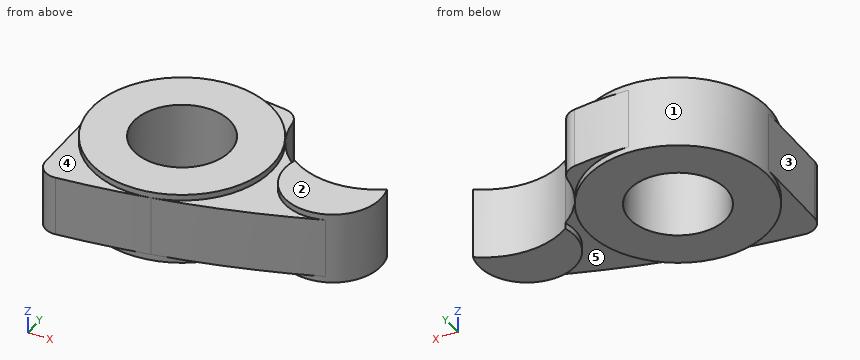
from build123d import *

# Parameters (mm, degrees)
SKETCH_1_R      = 15
SKETCH_1_R_2    = 8
EXTRUDE_1_DEPTH = 6
EXTRUDE_3_DEPTH = 6
EXTRUDE_4_DEPTH = 5


with BuildPart() as part:
    # Sketch 1 → Extrude 1 (new, symmetric)
    with BuildSketch(Plane.XY):
        Circle(SKETCH_1_R)
        Circle(SKETCH_1_R_2, mode=Mode.SUBTRACT)
    extrude(amount=EXTRUDE_1_DEPTH, both=True)



with BuildPart() as body_2:
    # Sketch 2 → Extrude 3 (new, symmetric)
    with BuildSketch(Plane.XY):
        with BuildLine():
            ThreePointArc((17.364190492, 2.386296955), (19.534557037, -5.841997366), (27.889014085, -7.460133888))
            ThreePointArc((27.889014085, -7.460133888), (32.219376902, -3.446824212), (32.617582381, 2.443857334))
            ThreePointArc((32.617582381, 2.443857334), (25, 0), (17.364190492, 2.386296955))
        make_face()
    extrude(amount=EXTRUDE_3_DEPTH, both=True)


with BuildPart() as part_1:
    add(part.part)

    add(body_2.part)  # Extrude 4 merges body 2
    # Sketch 2_4 → Extrude 4 (add, symmetric)
    with BuildSketch(Plane.XY):
        with BuildLine():
            ThreePointArc((15, 0), (11.593101986, -9.51840251), (2.920001822, -14.713041472))
            ThreePointArc((2.920001822, -14.713041472), (15.561957057, -11.62862528), (27.889014085, -7.460133888))
            ThreePointArc((27.889014085, -7.460133888), (19.534557037, -5.841997366), (17.364190492, 2.386296955))
            ThreePointArc((17.364190492, 2.386296955), (15.029800011, 4.466277015), (13.247787509, 7.035348329))
            ThreePointArc((13.247787509, 7.035348329), (14.555356619, 3.625133609), (15, 0))
        make_face()
        with BuildLine():
            ThreePointArc((2.920001822, -14.713041472), (-9.51840251, -11.593101986), (-15, 0))
            Line((-15, 0), (-15, -13.8873794))
            ThreePointArc((-15, -13.8873794), (-14.015653031, -16.10934764), (-11.708571429, -16.873190745))
            ThreePointArc((-11.708571429, -16.873190745), (-4.367649809, -15.973488812), (2.920001822, -14.713041472))
        make_face()
        with BuildLine():
            ThreePointArc((9.245195089, 14.463447909), (4.635046482, 14.946228489), (0, 15))
            ThreePointArc((0, 15), (7.728834811, 12.855547926), (13.247787509, 7.035348329))
            ThreePointArc((13.247787509, 7.035348329), (12.284448117, 9.358081475), (11.777275068, 11.820983737))
            ThreePointArc((11.777275068, 11.820983737), (10.960851201, 13.57305004), (9.245195089, 14.463447909))
        make_face()
    extrude(amount=EXTRUDE_4_DEPTH, both=True)


solid = part_1.part
Could you check a few things on this model? Use its own coordinates, in mm. Face numbers are marked on the shaded views. A direction names the side the tool comes from. Coordinates: 2 decimals unless noted, no trailing zeros. Order: outer loops, then holes, each group sorted by start corner. A loop starts at its lowest first (then second) coordinate and runs counter-clockwise, first axis right, second up.
Q1. Suppose I cut it at D-D on y = -12. Please give me the cut outline in (x, z).
Q2. Will these pins go through, and if not, where does the flat tip stop? pin 1 (2 mm diameter, centred on x = 14, y = -10, fed in from -Z); pin 2 (1 mm diameter, centred on y = 7, z = -3.5, fed in from +X); pin 3 (3 mm diameter, centred on x = 28, z = 4.5, fed in from -Y).
Q3. Suppose I cut it at C-C on x = 11. Please give me the cut outline in (y, z), and give its area (3 significant figures).
Q4. Which directions (+Z, -Z, +X, -X, +Y, -Y) give clear straight access to the entire face, cutting with the end or side of a thin tool? Please do the marked faces 1 and 2.
Q5. Thinking about a two-plate mould opening in X: for the marked faces 3, 4 and 5, which applies, released by +X, released by -X, zero draft, split by the parting line, or undercut?
Q6. Suppose I cut it at B-B on z = -1.25. Please give me the cut outline in (x, y), and give its area (3 significant figures).
Q7. Suppose I cut it at A-A on y = 4.5. Please give me the cut outline in (x, z), and give its area (3 significant figures).
Q8. Please list where these lines run through material, in increasing order: L1, parallel to Z at x = 8.5, y = 14.5; L2, parallel to Y at x = 0, z = -3; L3, parallel to Y at x = 6.5, z = 4.
Answer:
1. outline: (-15, -5) - (-9, -5) - (-9, -6) - (9, -6) - (9, -5) - (14.26, -5) - (14.26, 5) - (9, 5) - (9, 6) - (-9, 6) - (-9, 5) - (-15, 5) - close
2. pin 1: stops at z = -5
2. pin 2: stops at x = 13.55
2. pin 3: stops at y = -7.99
3. outline: (-12.88, -5) - (-10.2, -5) - (-10.2, -6) - (10.2, -6) - (10.2, -5) - (13.53, -5) - (13.53, 5) - (10.2, 5) - (10.2, 6) - (-10.2, 6) - (-10.2, 5) - (-12.88, 5) - close
3. area: 305 mm2
4. face 1: none
4. face 2: +Z, +X, -X, +Y, -Y
5. face 3: released by -X
5. face 4: zero draft
5. face 5: undercut
6. outline: (-15, -13.89) arc R3 ccw to (-11.71, -16.87) arc R150 ccw to (27.89, -7.46) arc R8 ccw to (32.62, 2.44) arc R13.25 cw to (11.78, 11.82) arc R3 ccw to (9.25, 14.46) arc R50 ccw to (0, 15) arc R15 ccw to (-15, 0) - close; hole circle Ø16 at (0, 0)
6. area: 792 mm2
7. outline: (-14.31, -6) - (-6.61, -6) - (-6.61, 6) - (-14.31, 6) - close; (6.61, -6) - (14.31, -6) - (14.31, -5) - (15, -5) - (15, 5) - (14.31, 5) - (14.31, 6) - (6.61, 6) - close
7. area: 192 mm2
8. L1: z = -5 to 5
8. L2: y = -15.26 to -8, 8 to 15
8. L3: y = -13.96 to -4.66, 4.66 to 14.8
